The listing builds one solid part. Answer for the finished solid, in the listing's coordinates (mm). A direction names the side the tool comes from. Coordinates: 2 decimals unless noted, no trailing zeros. Write each loop counter-clockwise with the first axis right and the second up, starting at its lowest first coordinate (ties: lowest second). Pieces come first, ordered by that corner, then holes.
from build123d import *

# Parameters (mm, degrees)
CROQUIS1_R              = 0.79375
CROQUIS1_R_2            = 1.5875
CROQUIS1_W              = 11.8
CROQUIS1_H              = 22.2
SALIENTE_EXTRUIR1_DEPTH = 3.175
CROQUIS2_R              = 1.5875
CORTAR_EXTRUIR1_DEPTH   = 3.175
CROQUIS3_W              = 10
CROQUIS3_H              = 4.7625
SALIENTE_EXTRUIR2_DEPTH = 3.175


with BuildPart() as part:
    # Croquis1 → Saliente-Extruir1 (new body)
    with BuildSketch(Plane(origin=(0, 0, 0), x_dir=(1, 0, 0), z_dir=(0, 1, 0))):
        with BuildLine():
            Line((8.713785816, 43.568929081), (0, 0))
            Line((0, 0), (60, 0))
            Line((60, 0), (51.286214184, 43.568929081))
            ThreePointArc((51.286214184, 43.568929081), (48.513480023, 48.186737131), (43.441568778, 50))
            Line((43.441568778, 50), (16.558431222, 50))
            ThreePointArc((16.558431222, 50), (11.486519977, 48.186737131), (8.713785816, 43.568929081))
        make_face()
        with Locations((39.75, 5.3)):
            Circle(CROQUIS1_R, mode=Mode.SUBTRACT)
        with Locations((39.75, 32.5)):
            Circle(CROQUIS1_R, mode=Mode.SUBTRACT)
        with Locations((20.25, 14)):
            Circle(CROQUIS1_R_2, mode=Mode.SUBTRACT)
        with Locations((24.75, 44)):
            Circle(CROQUIS1_R_2, mode=Mode.SUBTRACT)
        with Locations((35.25, 44)):
            Circle(CROQUIS1_R_2, mode=Mode.SUBTRACT)
        with Locations((39.75, 18.9)):
            Rectangle(CROQUIS1_W, CROQUIS1_H, mode=Mode.SUBTRACT)
    extrude(amount=SALIENTE_EXTRUIR1_DEPTH)

    # Croquis2 → Cortar-Extruir1 (cut)
    with BuildSketch(Plane(origin=(0, 3.175, 0), x_dir=(1, 0, 0), z_dir=(0, 1, 0))):
        with Locations((30, 35)):
            Circle(CROQUIS2_R)
        with Locations((6.099019514, 5)):
            Circle(CROQUIS2_R)
        with Locations((53.900980486, 5)):
            Circle(CROQUIS2_R)
        with BuildLine():
            Line((53.900980486, 0), (60, 0))
            Line((60, 0), (58.803883865, 5.980580676))
            ThreePointArc((58.803883865, 5.980580676), (57.767691193, 1.830055472), (53.900980486, 0))
        make_face()
        with BuildLine():
            Line((1.196116135, 5.980580676), (0, 0))
            Line((0, 0), (6.099019514, 0))
            ThreePointArc((6.099019514, 0), (2.232308807, 1.830055472), (1.196116135, 5.980580676))
        make_face()
    extrude(amount=-CORTAR_EXTRUIR1_DEPTH, mode=Mode.SUBTRACT)

    # Croquis3 → Saliente-Extruir2 (add)
    with BuildSketch(Plane(origin=(0, 3.175, 0), x_dir=(1, 0, 0), z_dir=(0, 1, 0))):
        with Locations((20, -2.38125)):
            Rectangle(CROQUIS3_W, CROQUIS3_H)
        with Locations((40, -2.38125)):
            Rectangle(CROQUIS3_W, CROQUIS3_H)
    extrude(amount=-SALIENTE_EXTRUIR2_DEPTH)


solid = part.part
1. Section B-B on z = -32.5 is taken. Give the vertices of the cut face in (x, y) (3 decimals), then the cut area to 3 significant figures.
Results found:
outline: (6.5, 0) - (38.956, 0) - (38.956, 3.175) - (6.5, 3.175) - close; (40.544, 0) - (53.5, 0) - (53.5, 3.175) - (40.544, 3.175) - close
area: 144 mm2
2. A tool of negligible diameter and unlimited length cuts with its end or side. For faces 5 (the flat face through (10, 2, 0)), 6 (the flat face through (5, 2, -25)), 7 (the flat face through (35, 2, 2)), 8 (the flat face through (45.65, 2, -19)), from which of +Z, -Z, +X, -X, +Y, -Y can it reach the whole face along a straight path? Write none if from no direction.
Results found:
face 5: +Z, -X, +Y, -Y
face 6: -Z, -X, +Y, -Y
face 7: +Z, +Y, -Y
face 8: +Y, -Y
3. Section D-D on z = -1 is taken. Give the vertices of the cut face in (x, y) (3 decimals).
Results found:
outline: (3.099, 0) - (56.901, 0) - (56.901, 3.175) - (3.099, 3.175) - close
4. Find the intervals of material crossed by L1, parallel to X at y = 1.25, z = -44; L2, parallel to X at y = 0.25, z = -43; L3, parallel to X at y = 2.25, z = 2, in increasing order.
Results found:
L1: x = 8.81 to 23.16, 26.34 to 33.66, 36.84 to 51.19
L2: x = 8.6 to 23.52, 25.98 to 34.02, 36.48 to 51.4
L3: x = 15 to 25, 35 to 45
5. For a pull along X with two mould halves and no side action, classify faces 1 (the flat face through (15, 2, 2)), 2 (the flat face through (30, 2, 0)), 3 (the flat face through (30, 2, -50)), 4 (the cylindrical face through (7.565, 1.61, -4.392)) as pulls with the +X half, pulls with the -X half, needs draft (parallel to the pull), parting line crosses it, or undercut.
Results found:
face 1: pulls with the -X half
face 2: undercut
face 3: needs draft
face 4: undercut
6. Flat-ended cylindrical pins translate along their axes: P1, Ø1, axis at y = 1, z = -24, coming from the +X side; P2, Ø2.5, axis at x = 24.75, z = -44, coming from the +Y side; P3, Ø1.6, axis at y = 1.5, z = 1.5, coming from the -X side; P4, Ø1.6, axis at y = 2, z = -22.5, coming from the +X side. Find the tip coordinate at first contact, or state that the pin passes through.
Results found:
P1: stops at x = 55.3
P2: passes through
P3: stops at x = 15
P4: stops at x = 55.66
7. Section A-A on x = 20.25 is taken. Give the vertices of the cut face in (y, z) (1 decimal), then the cut area to 3 significant figures.
Results found:
outline: (0, -50) - (3.2, -50) - (3.2, -15.6) - (0, -15.6) - close; (0, -12.4) - (3.2, -12.4) - (3.2, 4.8) - (0, 4.8) - close
area: 164 mm2
8. Section C-C on z = -14 is taken. State how many separate pieces and enclosed holes the cut face has, then the cut area to 3 significant figures.
Results found:
separate pieces: 3
enclosed holes: 0
area: 125 mm2
